Input: part model. Units: mm. Frame: model coordinates. A direction names the side the tool comes from. Coordinates: 2 decimals unless noted, no trailing zeros. Loops run counter-clockwise (first coordinate to the right, second up) from the corner with the lowest first, then second, coordinate; pieces in that order, holes last. Notation, with made-up numbers: (-10, 44.25) -> (34, 44.25) arc R7 ccw to (34, 50.25) -> close; hole circle Ø8 at (12.25, 25.25). An arc over 180 degrees is marked (long way). Answer as a JSON object with one key per item and string values.
from build123d import *

# Parameters (mm, degrees)
SKETCH_1_R      = 2.5
EXTRUDE_1_DEPTH = 40


with BuildPart() as part:
    # 草图1 → 凸台-拉伸1 (new body)
    with BuildSketch(Plane.XY):
        with BuildLine():
            Line((1604.394788332, 627.726005938), (1604.394788332, 644.726005938))
            ThreePointArc((1604.394788332, 644.726005938), (1603.955448504, 645.78666611), (1602.894788332, 646.226005938))
            Line((1602.894788332, 646.226005938), (1597.994788332, 646.226005938))
            Line((1597.994788332, 646.226005938), (1597.994788332, 645.926005938))
            ThreePointArc((1597.994788332, 645.926005938), (1597.936209689, 645.784584582), (1597.794788332, 645.726005938))
            Line((1597.794788332, 645.726005938), (1597.494788332, 645.726005938))
            Line((1597.494788332, 645.726005938), (1597.494788332, 644.726005938))
            ThreePointArc((1597.494788332, 644.726005938), (1597.582656298, 644.513873904), (1597.794788332, 644.426005938))
            Line((1597.794788332, 644.426005938), (1599.594788332, 644.426005938))
            ThreePointArc((1599.594788332, 644.426005938), (1599.806920367, 644.338137973), (1599.894788332, 644.126005938))
            Line((1599.894788332, 644.126005938), (1599.894788332, 642.786005938))
            Line((1599.894788332, 642.786005938), (1597.674128161, 640.565345767))
            ThreePointArc((1597.674128161, 640.565345767), (1597.187493137, 640.24018664), (1596.613467989, 640.126005938))
            Line((1596.613467989, 640.126005938), (1592.176108676, 640.126005938))
            ThreePointArc((1592.176108676, 640.126005938), (1591.602083527, 640.24018664), (1591.115448504, 640.565345767))
            Line((1591.115448504, 640.565345767), (1588.894788332, 642.786005938))
            Line((1588.894788332, 642.786005938), (1588.894788332, 644.126005938))
            ThreePointArc((1588.894788332, 644.126005938), (1588.982656298, 644.338137973), (1589.194788332, 644.426005938))
            Line((1589.194788332, 644.426005938), (1590.994788332, 644.426005938))
            ThreePointArc((1590.994788332, 644.426005938), (1591.206920367, 644.513873904), (1591.294788332, 644.726005938))
            Line((1591.294788332, 644.726005938), (1591.294788332, 645.726005938))
            Line((1591.294788332, 645.726005938), (1590.994788332, 645.726005938))
            ThreePointArc((1590.994788332, 645.726005938), (1590.853366976, 645.784584582), (1590.794788332, 645.926005938))
            Line((1590.794788332, 645.926005938), (1590.794788332, 646.226005938))
            Line((1590.794788332, 646.226005938), (1585.894788332, 646.226005938))
            ThreePointArc((1585.894788332, 646.226005938), (1584.834128161, 645.78666611), (1584.394788332, 644.726005938))
            Line((1584.394788332, 644.726005938), (1584.394788332, 627.726005938))
            ThreePointArc((1584.394788332, 627.726005938), (1584.834128161, 626.665345767), (1585.894788332, 626.226005938))
            Line((1585.894788332, 626.226005938), (1602.894788332, 626.226005938))
            ThreePointArc((1602.894788332, 626.226005938), (1603.955448504, 626.665345767), (1604.394788332, 627.726005938))
        make_face()
        with Locations((1594.394788332, 636.226005938)):
            Circle(SKETCH_1_R, mode=Mode.SUBTRACT)
        with BuildLine():
            Line((1598.734128161, 639.505345767), (1600.954788332, 641.726005938))
            Line((1600.954788332, 641.726005938), (1602.294788332, 641.726005938))
            ThreePointArc((1602.294788332, 641.726005938), (1602.506920367, 641.638137973), (1602.594788332, 641.426005938))
            Line((1602.594788332, 641.426005938), (1602.594788332, 631.026005938))
            ThreePointArc((1602.594788332, 631.026005938), (1602.506920367, 630.813873904), (1602.294788332, 630.726005938))
            Line((1602.294788332, 630.726005938), (1600.954788332, 630.726005938))
            Line((1600.954788332, 630.726005938), (1598.734128161, 632.94666611))
            ThreePointArc((1598.734128161, 632.94666611), (1598.408969034, 633.433301133), (1598.294788332, 634.007326282))
            Line((1598.294788332, 634.007326282), (1598.294788332, 638.444685595))
            ThreePointArc((1598.294788332, 638.444685595), (1598.408969034, 639.018710743), (1598.734128161, 639.505345767))
        make_face(mode=Mode.SUBTRACT)
        with BuildLine():
            Line((1586.194788332, 631.026005938), (1586.194788332, 641.426005938))
            ThreePointArc((1586.194788332, 641.426005938), (1586.282656298, 641.638137973), (1586.494788332, 641.726005938))
            Line((1586.494788332, 641.726005938), (1587.834788332, 641.726005938))
            Line((1587.834788332, 641.726005938), (1590.055448504, 639.505345767))
            ThreePointArc((1590.055448504, 639.505345767), (1590.380607631, 639.018710743), (1590.494788332, 638.444685595))
            Line((1590.494788332, 638.444685595), (1590.494788332, 634.007326282))
            ThreePointArc((1590.494788332, 634.007326282), (1590.380607631, 633.433301133), (1590.055448504, 632.94666611))
            Line((1590.055448504, 632.94666611), (1587.834788332, 630.726005938))
            Line((1587.834788332, 630.726005938), (1586.494788332, 630.726005938))
            ThreePointArc((1586.494788332, 630.726005938), (1586.282656298, 630.813873904), (1586.194788332, 631.026005938))
        make_face(mode=Mode.SUBTRACT)
        with BuildLine():
            Line((1599.594788332, 628.026005938), (1589.194788332, 628.026005938))
            ThreePointArc((1589.194788332, 628.026005938), (1588.982656298, 628.113873904), (1588.894788332, 628.326005938))
            Line((1588.894788332, 628.326005938), (1588.894788332, 629.666005938))
            Line((1588.894788332, 629.666005938), (1591.115448504, 631.88666611))
            ThreePointArc((1591.115448504, 631.88666611), (1591.602083527, 632.211825237), (1592.176108676, 632.326005938))
            Line((1592.176108676, 632.326005938), (1596.613467989, 632.326005938))
            ThreePointArc((1596.613467989, 632.326005938), (1597.187493137, 632.211825237), (1597.674128161, 631.88666611))
            Line((1597.674128161, 631.88666611), (1599.894788332, 629.666005938))
            Line((1599.894788332, 629.666005938), (1599.894788332, 628.326005938))
            ThreePointArc((1599.894788332, 628.326005938), (1599.806920367, 628.113873904), (1599.594788332, 628.026005938))
        make_face(mode=Mode.SUBTRACT)
    extrude(amount=EXTRUDE_1_DEPTH)


solid = part.part
1. Section query B-B (x = 1595). Return loops of the section in (y, z).
Reply:
{"outline": "(626.23, 0) -> (628.03, 0) -> (628.03, 40) -> (626.23, 40) -> close; (632.33, 0) -> (633.8, 0) -> (633.8, 40) -> (632.33, 40) -> close; (638.65, 0) -> (640.13, 0) -> (640.13, 40) -> (638.65, 40) -> close"}
2. Section query A-A (y = 629.25). Return loops of the section in (x, z), plus the area to 3 significant figures.
Reply:
{"outline": "(1584.39, 0) -> (1588.89, 0) -> (1588.89, 40) -> (1584.39, 40) -> close; (1599.89, 0) -> (1604.39, 0) -> (1604.39, 40) -> (1599.89, 40) -> close", "area": "360 mm2"}
3. Section query C-C (y = 637.25). Return loops of the section in (x, z).
Reply:
{"outline": "(1584.39, 0) -> (1586.19, 0) -> (1586.19, 40) -> (1584.39, 40) -> close; (1590.49, 0) -> (1592.11, 0) -> (1592.11, 40) -> (1590.49, 40) -> close; (1596.68, 0) -> (1598.29, 0) -> (1598.29, 40) -> (1596.68, 40) -> close; (1602.59, 0) -> (1604.39, 0) -> (1604.39, 40) -> (1602.59, 40) -> close"}
4. Line query: line 1 along X through (y, z) = (639.5, 34); line 2 along X through (y, z) = (635.75, 37); line 3 along X through (y, z) = (633.25, 3). Output: solid intervals per line, ascending.
Reply:
{"line 1": "x = 1584.39 to 1586.19, 1590.06 to 1598.73, 1602.59 to 1604.39", "line 2": "x = 1584.39 to 1586.19, 1590.49 to 1591.94, 1596.85 to 1598.29, 1602.59 to 1604.39", "line 3": "x = 1584.39 to 1586.19, 1590.29 to 1598.5, 1602.59 to 1604.39"}
5. Section query D-D (z = 37). Count the separate pieces of the cut face and the enclosed holes in it, plus the area to 3 significant figures.
Reply:
{"separate pieces": "1", "enclosed holes": "4", "area": "206 mm2"}
6. Pin query (flat end, axial travel): P1, Ø1, axis at x = 1596.5, z = 33.5, coming from the +Y side; P2, Ø2, axis at x = 1594, z = 27.5, coming from the +Y side. Return the tip coordinate at first contact, or that it passes through.
Reply:
{"P1": "stops at y = 640.18", "P2": "stops at y = 640.13"}
7. Access query for faces 5 (the face through (1597.495, 645, 20)), 6 (the face through (1592, 634, 40)), 7 (the face through (1602, 630.726, 20)). Directions: +Z, -Z, +X, -X, +Y, -Y. A direction counts if a zero-diameter tool reaches every point of the face in a straight line with its end or side. Return the directions, or none.
Reply:
{"face 5": "+Z, -Z, +Y", "face 6": "+Z, +X, -X, +Y, -Y", "face 7": "+Z, -Z"}
8. Mould query, pull axis Y, two halves, no side actions, for faces 1 (the face through (1594, 632.326, 20)), 2 (the face through (1584.8, 626.7, 19.7)), 3 (the face through (1590.384, 633.441, 19.72)), 4 (the face through (1594, 640.126, 20)). Classes: pulls with the +Y half, pulls with the -Y half, needs draft (parallel to the pull), parting line crosses it, or undercut.
Reply:
{"face 1": "undercut", "face 2": "pulls with the -Y half", "face 3": "undercut", "face 4": "pulls with the +Y half"}
